Autodesk Inventor part; units mm, degrees
ref_plane "YZ Plane" through (0, 0, 0) normal (1, 0, 0) x (0, 1, 0)
ref_plane "XZ Plane" through (0, 0, 0) normal (0, 1, 0) x (-1, 0, 0)
ref_plane "XY Plane" through (0, 0, 0) normal (0, 0, 1) x (1, 0, 0)
sketch "スケッチ1" plane through (0, 0, 0) normal (0, 0, 1) x (1, 0, 0)
  line L0 (0, -5.7735) -> (-5, -2.8868)
  line L1 (-5, -2.8868) -> (-5, 2.8868)
  line L2 (-5, 2.8868) -> (0, 5.7735)
  line L3 (0, 5.7735) -> (5, 2.8868)
  line L4 (5, 2.8868) -> (5, -2.8868)
  line L5 (5, -2.8868) -> (0, -5.7735)
  circle A0 centre (0, 0) radius 22.5
  circle A1 centre (0, 0) radius 20.9
  dimension "HUB_D" = 10
  dimension "DIA" = 45
  dimension "RIM_THIN" = 1.6
extrude "ハブ＆リム" add sketch "スケッチ1" along normal blind 10
sketch "スケッチ2" plane through (0, 0, 10) normal (0, 0, 1) x (1, 0, 0)
  line L0 (-0.8, 0) -> (0.8, 0)
  line L1 (0.8, 0) -> (0.8, 20.9)
  line L2 (0.8, 20.9) -> (-0.8, 20.9)
  line L3 (-0.8, 20.9) -> (-0.8, 0)
  line L4 (0, 0) -> (0, 25.5289) construction
  circle A0 centre (0, 0) radius 20.9 construction
  point P0 (0, 20.9)
  dimension "SPOKE_THIN" = 1.6
extrude "スポーク" add sketch "スケッチ2" against normal up to surface (10 mm away)
pattern_circular "円形状パターン1" count 6 over 360 about axis through (0, 0, -10) along (0, 0, 1) of "スポーク"
sketch "スケッチ3" plane through (0, 0, 10) normal (0, 0, 1) x (1, 0, 0)
  line L0 (-2.5, 1.525) -> (2.5, 1.525)
  line L1 (2.5, 1.525) -> (2.5, -1.525)
  line L2 (2.5, -1.525) -> (-2.5, -1.525)
  line L3 (-2.5, -1.525) -> (-2.5, 1.525)
  point P0 (0, 0)
  point P1 (0, 1.525)
  point P2 (2.5, 0)
  dimension "d11" = 5
  dimension "d12" = 3.05
extrude "押し出し3" cut sketch "スケッチ3" against normal through all
properties part number "Wheel-D45B"
Read the model definition and answer for the solid it produces. Units are mm, in the model's axes. A direction names the side the tool comes from. Round coordinates to 2 decimals unless told otherwise and drop trailing zeros. Write each loop counter-clockwise with the first axis right and the second up, starting at its lowest first coordinate (ties: lowest second). Pieces come first, ordered by that corner, then holes. Notation, with made-up numbers: (80.25, -32) - (130.25, -32) arc R21 cw to (130.25, -10) - close; hole circle Ø9 at (74, -13). An arc over 180 degrees is marked (long way). One line per question, with ' | ' between items. Start each with the question number.
1. Section A-A (x = 0) is taken. Determine the outline of the cut face in (y, z) (3 decimals), and give its area (4 significant figures).
2. For a pull along Y with two mould halves and no side action, classify faces 1 (the face through (0, -2, 0)), 2 (the face through (2.48, 4.34, 4.93)) as +Y half, -Y half, draft (parallel to the pull), parting line (faces both ways), or undercut.
3. Each of these flat-tipped pins is pushed along its axis until it touches: pin 1 (2 mm diameter, centred on x = 15.5, z = 4.5, fed in from +Y); pin 2 (5 mm diameter, centred on y = -12.5, z = 6, fed in from +X); pin 3 (5 mm diameter, centred on y = -15.5, z = 8, fed in from -X). Where does it stop, or does it pass through?
4. Section B-B (z = 7) is taken. Give the number of separate pieces and of enclosed holes in the cut face, and give its area (3 significant figures).
5. Find the intervals of material crossed by probe 1 along X at (y, z) = (0.5, 9.5); probe 2 along Y at (x, z) = (-6, 4.5); probe 3 along Y at (x, z) = (-3, 1.5), in increasing order. Write a range as [from, to].
6. Section C-C (y = 0) is taken. Determine the outline of the cut face in (x, z), and give its area (3 significant figures).
7. For faces 3 (the face through (10.57, -18.03, 4.93)), 4 (the face through (3, 2, 10)), determine the directions among +Z, -Z, +X, -X, +Y, -Y from which every point of the face is accessible in a straight line to the end or side of a thin tool.
8. Section D-D (x = 13) is taken. Determine the outline of the cut face in (y, z), and give its area (3 significant figures).
Filled in:
1) outline: (-22.5, 0) - (-1.525, 0) - (-1.525, 10) - (-22.5, 10) - close; (1.525, 0) - (22.5, 0) - (22.5, 10) - (1.525, 10) - close | area: 419.5 mm²
2) face 1: draft | face 2: undercut
3) pin 1: y = 17.2 | pin 2: x = 20.16 | pin 3: x = -18.36
4) separate pieces: 1 | enclosed holes: 7 | area: 437 mm²
5) probe 1: [-22.49, -20.89], [-5, -2.5], [2.5, 5], [20.89, 22.49] | probe 2: [-21.69, -20.02], [-4.39, -2.54], [2.54, 4.39], [20.02, 21.69] | probe 3: [-22.3, -20.68], [-4.04, 4.04], [20.68, 22.3]
6) outline: (-22.5, 0) - (-20.9, 0) - (-20.9, 10) - (-22.5, 10) - close; (-5, 0) - (-2.5, 0) - (-2.5, 10) - (-5, 10) - close; (2.5, 0) - (5, 0) - (5, 10) - (2.5, 10) - close; (20.9, 0) - (22.5, 0) - (22.5, 10) - (20.9, 10) - close | area: 82.0 mm²
7) face 3: +Z, -Z | face 4: +Z, +X, -X, +Y, -Y
8) outline: (-18.36, 0) - (-16.36, 0) - (-16.36, 10) - (-18.36, 10) - close; (-8.43, 0) - (-6.58, 0) - (-6.58, 10) - (-8.43, 10) - close; (6.58, 0) - (8.43, 0) - (8.43, 10) - (6.58, 10) - close; (16.36, 0) - (18.36, 0) - (18.36, 10) - (16.36, 10) - close | area: 76.9 mm²
